For this review, use the dimensioned drawing (mm, ordinates from the lowest corner) and the shaded views. Coordinates: 2 decimals unless noted, no trailing zeros. Loops run counter-clockwise (first coordinate to the right, second up) from the corner with the lowest first, then second, coordinate; pieces in that order, holes last. Notation, with made-up numbers: (45.5, 37) - (59.5, 37) arc R21 ccw to (59.5, 71) - close; hole circle Ø2 at (-38, -40). An arc over 180 degrees is marked (long way). Answer in a Markdown table with one row per item. Add a question column.
(1) We need section D-D on y = 7.25. Write out the cut boundary in (x, z), plus the area to 3 significant figures.
(2) We need section A-A on z = 121. Write out the cut boundary in (x, y), plus the area to 3 significant figures.
(3) We need section B-B on x = 95. Write out the cut boundary in (y, z).
(4) For line 1 along Z through (x, y) = (95, 7.5); line 2 along X through (y, z) = (6.5, 121); line 3 along Z through (x, y) = (250, 7.5), list the stretches that pass through material, from the lowest coordinate up.
(5) For P1, Ø21, axis at x = 95, z = 431, coming from the +Y side, flat-tipped, find the tip position at first contact; note if it passes through.
(6) We need section C-C on x = 250. Write out the cut boundary in (y, z), plus the area to 3 significant figures.
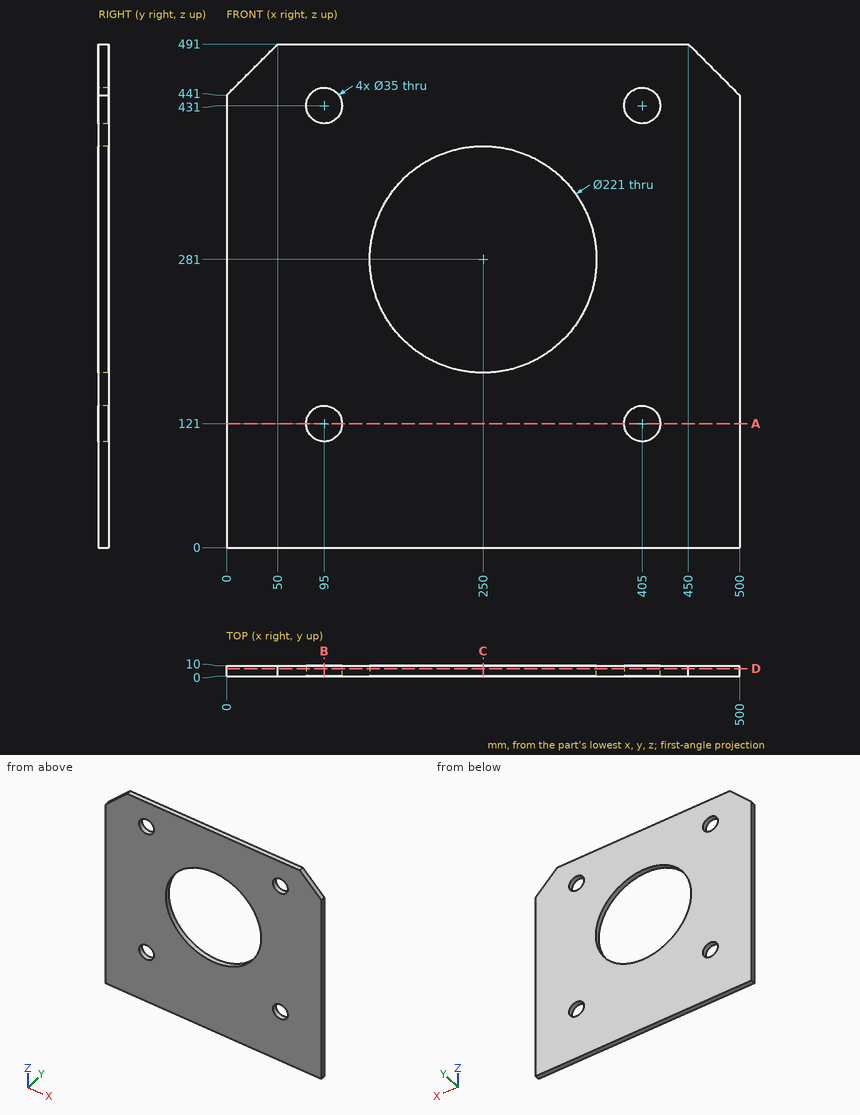
Outcome:
| question | item | result |
|---|---|---|
| 1 | outline | (0, 0) - (500, 0) - (500, 441) - (450, 491) - (50, 491) - (0, 441) - close; hole circle Ø35 at (95, 121); hole circle Ø35 at (95, 431); hole circle Ø221 at (250, 281); hole circle Ø35 at (405, 121); hole circle Ø35 at (405, 431) |
| 1 | area | 201,000 mm² |
| 2 | outline | (0, 0) - (77.5, 0) - (77.5, 10) - (0, 10) - close; (112.5, 0) - (387.5, 0) - (387.5, 10) - (112.5, 10) - close; (422.5, 0) - (500, 0) - (500, 10) - (422.5, 10) - close |
| 2 | area | 4,300 mm² |
| 3 | outline | (0, 0) - (10, 0) - (10, 103.5) - (0, 103.5) - close; (0, 138.5) - (10, 138.5) - (10, 413.5) - (0, 413.5) - close; (0, 448.5) - (10, 448.5) - (10, 491) - (0, 491) - close |
| 4 | line 1 | 0 to 103.5, 138.5 to 413.5, 448.5 to 491 |
| 4 | line 2 | 0 to 77.5, 112.5 to 387.5, 422.5 to 500 |
| 4 | line 3 | 0 to 170.5, 391.5 to 491 |
| 5 | P1 | through |
| 6 | outline | (0, 0) - (10, 0) - (10, 170.5) - (0, 170.5) - close; (0, 391.5) - (10, 391.5) - (10, 491) - (0, 491) - close |
| 6 | area | 2,700 mm² |
